Autodesk Inventor part; units mm, degrees
ref_plane "YZ Plane" through (0, 0, 0) normal (1, 0, 0) x (0, 1, 0)
ref_plane "XZ Plane" through (0, 0, 0) normal (0, 1, 0) x (-1, 0, 0)
ref_plane "XY Plane" through (0, 0, 0) normal (0, 0, 1) x (1, 0, 0)
sketch "Esboço1" plane through (0, 0, 0) normal (0, 1, 0) x (-1, 0, 0)
  line L0 (17.5, -25) -> (-17.5, -25)
  line L1 (-17.5, -25) -> (-17.5, 25)
  line L2 (-17.5, 25) -> (17.5, 25)
  line L3 (17.5, 25) -> (17.5, -25)
  line L4 (17.5, -25) -> (-17.5, 25) construction
  line L5 (-17.5, -25) -> (17.5, 25) construction
  point P0 (0, 0)
  dimension "d0" = 35
  dimension "d1" = 50
extrude "Extrusão1" add sketch "Esboço1" along normal blind 60
chamfer "Chanfro1" distance 20 angle 60 1 edges at (0, 60, 25) measured on face at (5.8333, 60, 8.3333)
sketch "Esboço2" plane through (17.5, 0, -25) normal (0, 0, -1) x (-1, 0, 0)
  line L0 (0, 60) -> (15, 60)
  line L1 (15, 60) -> (15, 40)
  line L2 (15, 40) -> (0, 40)
  line L3 (0, 40) -> (0, 60)
  line L4 (35, 0) -> (35, 60)
  line L5 (0, 0) -> (35, 0)
  point P0 (17.5, 0)
  dimension "d7" = 20
  dimension "d8" = 40
extrude "Extrusão2" cut sketch "Esboço2" against normal through all
properties part number "3D Model"
Geometry check sheet. Reference: the model listing, model coordinates, mm. A direction names the side the tool comes from. Round coordinates to 2 decimals unless told otherwise and drop trailing zeros. Write each loop counter-clockwise with the first axis right and the second up, starting at its lowest first coordinate (ties: lowest second). Pieces come first, ordered by that corner, then holes. Notation, with made-up numbers: (49.25, 41) - (91.25, 41) arc R13 ccw to (91.25, 53) - close; hole circle Ø5 at (45.25, 31.5). An arc over 180 degrees is marked (long way). One line per item, written item: value.
1. Depth check by flat-ended pin: pin 1 Ø10 at (y, z) = (46.5, -1) entering from +X; pin 2 Ø3 at (x, y) = (8, 40.5) entering from +Z. Enter the tip coordinate at first touch or a pass-through.
The answers:
pin 1: stops at x = 2.5
pin 2: stops at z = 17.12
2. Scan lines: L1, parallel to Y at x = 12, z = -21; L2, parallel to X at y = 54.5, z = -3; L3, parallel to Y at x = -1, z = 6.5. Record each from-to range of solid material in increasing order.
The answers:
L1: y = 0 to 40
L2: x = -17.5 to 2.5
L3: y = 0 to 57.4
3. Cross-section at D-D on x = -8.5. Record the boundary of the cut face in (y, z), and give its area (3 significant figures).
The answers:
outline: (0, -25) - (60, -25) - (60, 5) - (25.36, 25) - (0, 25) - close
area: 2,650 mm^2
4. Cross-section at B-B on x = 3.5. Record the boundary of the cut face in (y, z).
The answers:
outline: (0, -25) - (40, -25) - (40, 16.55) - (25.36, 25) - (0, 25) - close
5. Cross-section at C-C on y = 33.5. Record the boundary of the cut face in (x, z), and give its area (3 significant figures).
The answers:
outline: (-17.5, -25) - (17.5, -25) - (17.5, 20.3) - (-17.5, 20.3) - close
area: 1,590 mm^2
6. Set-up check for faces 1 (the face through (2.5, 50, -9)), 2 (the face through (0, 23, -25)): record each of +Z, -Z, +X, -X, +Y, -Y from which the full face is reachable in a straight line by a thin tool's end or side.
The answers:
face 1: +Z, -Z, +X, +Y
face 2: -Z, +X, -X, +Y, -Y
7. Cross-section at A-A on z = 0. Record the boundary of the cut face in (x, y), and give its area (3 significant figures).
The answers:
outline: (-17.5, 0) - (17.5, 0) - (17.5, 40) - (2.5, 40) - (2.5, 60) - (-17.5, 60) - close
area: 1,800 mm^2
